```python
from build123d import *
from build123d.topology import SkipClean

# Parameters (mm, degrees)
SKETCH_1_R               = 5
SKETCH_1_R_2             = 3.5
EXTRUDE_1_DEPTH          = 2
EXTRUDE_2_DEPTH          = 2
CUT_EXTRUDE_1_DEPTH      = 61.539243471
CUT_EXTRUDE_1_DEPTH_BACK = 61.539243471
EXTRUDE_3_DEPTH          = 0.25
EXTRUDE_4_DEPTH          = 2
CUT_EXTRUDE_START        = 1
CUT_EXTRUDE_2_DEPTH      = 63.641007782
CUT_EXTRUDE_3_DEPTH      = 61.641007782
CUT_EXTRUDE_3_DEPTH_BACK = 61.641007782
SKETCH_8_R               = 0.706141664
EXTRUDE_5_DEPTH          = 4.5


with BuildPart() as part:
    # 草图1 → 凸台-拉伸1 (new, symmetric)
    with BuildSketch(Plane(origin=(0, 0, 0), x_dir=(1, 0, 0), z_dir=(0, 1, 0))):
        with Locations(Location((0, 0, 0), (0, 0, 270))):
            Circle(SKETCH_1_R)
        with Locations(Location((0, 0, 0), (0, 0, 270))):
            Circle(SKETCH_1_R_2, mode=Mode.SUBTRACT)
    extrude(amount=EXTRUDE_1_DEPTH, both=True)

    # 草图3 → 凸台-拉伸2 (add, symmetric)
    with BuildSketch(Plane(origin=(0, 0, 0), x_dir=(1, 0, 0), z_dir=(0, 1, 0))):
        with BuildLine():
            ThreePointArc((-4.530759254, -2.114762536), (-2.959942563, -6.862777701), (-2.534847218, -11.845789545))
            Line((-2.534847218, -11.845789545), (-3.308166283, -35.931035681))
            ThreePointArc((-3.308166283, -35.931035681), (-4.349252604, -47.119849682), (-6.737299363, -58.100316528))
            ThreePointArc((-6.737299363, -58.100316528), (0, -53), (6.737299363, -58.100316528))
            ThreePointArc((6.737299363, -58.100316528), (4.349252604, -47.119849682), (3.308166283, -35.931035681))
            Line((3.308166283, -35.931035681), (2.534847218, -11.845789545))
            ThreePointArc((2.534847218, -11.845789545), (2.959942563, -6.862777701), (4.530759254, -2.114762536))
            ThreePointArc((4.530759254, -2.114762536), (0, -5), (-4.530759254, -2.114762536))
        make_face()
        with BuildLine():
            Line((-7, -60), (7, -60))
            ThreePointArc((7, -60), (0, -53), (-7, -60))
        make_face()
    extrude(amount=EXTRUDE_2_DEPTH, both=True)

    # 草图4 → 切除-拉伸1 (cut, two sides: drawn at the far end of the back side and taken through both)
    with BuildSketch(Plane(origin=(0, 2, 0), x_dir=(1, 0, 0), z_dir=(0, 1, 0)).offset(-CUT_EXTRUDE_1_DEPTH_BACK)):
        with BuildLine():
            Line((-3, -60), (3, -60))
            ThreePointArc((3, -60), (0, -57), (-3, -60))
        make_face()
    extrude(amount=CUT_EXTRUDE_1_DEPTH + CUT_EXTRUDE_1_DEPTH_BACK, mode=Mode.SUBTRACT)

    # 草图5 → 凸台-拉伸3 (add, symmetric)
    with SkipClean():  # the faces are left unmerged after this step: merging them gives an invalid solid
        with BuildSketch(Plane(origin=(0, 2, 0), x_dir=(1, 0, 0), z_dir=(0, 1, 0))):
            with BuildLine():
                Line((-3, -60), (-7, -60))
                ThreePointArc((-7, -60), (0, -53), (7, -60))
                Line((7, -60), (3, -60))
                ThreePointArc((3, -60), (0, -57), (-3, -60))
            make_face()
        extrude_3 = extrude(amount=EXTRUDE_3_DEPTH, both=True)

    # 镜向1: 凸台-拉伸3 across plane
    with SkipClean():  # the faces are left unmerged after this step: merging them gives an invalid solid
        add(extrude_3.mirror(Plane.ZX))

    # 草图6 → 凸台-拉伸4 (add, symmetric)
    with BuildSketch(Plane(origin=(0, 0, 0), x_dir=(1, 0, 0), z_dir=(0, 1, 0))):
        with BuildLine():
            Line((-8.501136679, -55.801748406), (-8.501136679, -60))
            Line((-8.501136679, -60), (-7, -60))
            ThreePointArc((-7, -60), (-6.934013828, -59.041119283), (-6.737299363, -58.100316528))
            ThreePointArc((-6.737299363, -58.100316528), (-4.907121304, -50.347633667), (-3.749679969, -42.466391834))
            ThreePointArc((-3.749679969, -42.466391834), (-5.3686221, -49.403716977), (-8.501136679, -55.801748406))
        make_face()
        with BuildLine():
            Line((8.501136679, -60), (7, -60))
            ThreePointArc((7, -60), (6.934013828, -59.041119283), (6.737299363, -58.100316528))
            ThreePointArc((6.737299363, -58.100316528), (4.907121304, -50.347633667), (3.749679969, -42.466391834))
            ThreePointArc((3.749679969, -42.466391834), (5.3686221, -49.403716977), (8.501136679, -55.801748406))
            Line((8.501136679, -55.801748406), (8.501136679, -60))
        make_face()
    extrude(amount=EXTRUDE_4_DEPTH, both=True)

    # 草图7 → 切除-拉伸2 (cut)
    with BuildSketch(Plane(origin=(0, 0, 0), x_dir=(1, 0, 0), z_dir=(0, 1, 0)).offset(CUT_EXTRUDE_START)):
        with BuildLine():
            Line((-2.032181597, -10.971248009), (-2.792905901, -34.66422669))
            ThreePointArc((-2.792905901, -34.66422669), (0, -35.636501302), (2.792905901, -34.66422669))
            Line((2.792905901, -34.66422669), (2.032181597, -10.971248009))
            ThreePointArc((2.032181597, -10.971248009), (0, -9.921815328), (-2.032181597, -10.971248009))
        make_face()
    cut_extrude_2 = extrude(amount=CUT_EXTRUDE_2_DEPTH, mode=Mode.SUBTRACT)

    # 镜向2: 切除-拉伸2 across plane
    add(cut_extrude_2.mirror(Plane.ZX), mode=Mode.SUBTRACT)

    # 草图8 → 切除-拉伸3 (cut, two sides: drawn at the far end of the back side and taken through both)
    with BuildSketch(Plane.XY.offset(-CUT_EXTRUDE_3_DEPTH_BACK)):
        with Locations((-6.917679895, 0.156331749)):
            Circle(SKETCH_8_R)
        with Locations((6.917679895, 0.156331749)):
            Circle(SKETCH_8_R)
    extrude(amount=CUT_EXTRUDE_3_DEPTH + CUT_EXTRUDE_3_DEPTH_BACK, mode=Mode.SUBTRACT)

    # 草图11 → 凸台-拉伸5 (add)
    with BuildSketch(Plane(origin=(0, 2.25, 0), x_dir=(1, 0, 0), z_dir=(0, 1, 0))):
        with BuildLine():
            Line((8.501136679, -64.198251594), (8.501136679, -60))
            Line((8.501136679, -60), (3, -60))
            ThreePointArc((3, -60), (0, -63), (-3, -60))
            Line((-3, -60), (-8.501136679, -60))
            Line((-8.501136679, -60), (-8.501136679, -64.198251594))
            ThreePointArc((-8.501136679, -64.198251594), (-8.066557797, -64.898765683), (-7.650409709, -65.61038325))
            ThreePointArc((-7.650409709, -65.61038325), (0, -69.487105403), (7.650409709, -65.61038325))
            ThreePointArc((7.650409709, -65.61038325), (8.066557797, -64.898765683), (8.501136679, -64.198251594))
        make_face()
    extrude(amount=-EXTRUDE_5_DEPTH)


solid = part.part
```
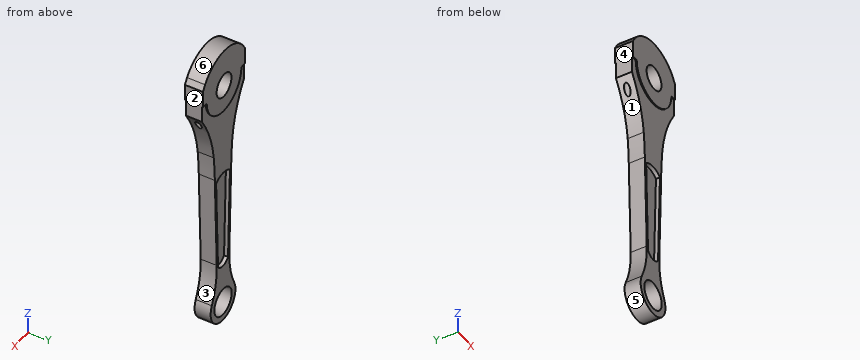
The model under review builds one solid part; all positions refer to its coordinate system, in mm. Face numbers are marked on the shaded views. A direction names the side the tool comes from. Give positions to 0.01 mm unless a question says otherwise; leave off trailing zeros. Write each loop counter-clockwise with the first axis right and the second up, starting at its lowest first coordinate (ties: lowest second). Pieces come first, ordered by that corner, then holes.
(1) To check wall thickness, follow L1, parallel to Z at x = 0.25, y = 1.35; L2, parallel to X at y = 1, z = 60; L3, parallel to X at y = -0.35, z = 0. State the ranges of each line that lie inside material, in increasing order.
(2) Tool access review of the marked faces 1, 2 and 3: name each direction out of +Z, -Z, +X, -X, +Y, -Y from which nothing blocks a thin tool from reaching the whole face with its end or side.
(3) Consider section D-D, the plane z = 41. Give the boundary of the cut face in (x, y), and give its area (3 significant figures).
(4) The part is to be moulded in two halves that separate along Z. For the marked faces 4, 5 and 6, say which applies: released by +Z, released by -Z, zero draft, split by the parting line, or undercut.
(5) Consider section B-B, the plane z = 0. Give the boundary of the cut face in (x, y), and give its area (3 significant figures).
(6) For P1, Ø3, axis at x = -0.5, z = 28.5, coming from the +Y side; P2, Ø1.3, axis at x = -6.92, y = 0.16, coming from the +Z side; P3, Ø1.6, axis at x = 7, y = 0, coming from the -Z side; P4, Ø5.5, axis at x = 0, z = 0, coming from the +Y side, all flat-tipped, find the tip position at first contact; note any pin that passes through.
(7) Consider section A-A, the plane x = 0. Give the boundary of the cut face in (y, z).
(8) Consider section C-C, the plane z = 13.5. Give the boundary of the cut face in (x, y).
Returned:
1. L1: z = -4.99 to -3.49, 3.49 to 9.93, 35.63 to 57.01, 62.99 to 69.48
1. L2: x = -8.5 to -3, 3 to 8.5
1. L3: x = -5 to -3.5, 3.5 to 5
2. face 1: -X, +Y, -Y
2. face 2: +Z, -Z, +X, +Y, -Y
2. face 3: +X, +Y, -Y
3. outline: (-3.61, -2) - (3.61, -2) - (3.61, 2) - (-3.61, 2) - close
3. area: 28.9 mm2
4. face 4: zero draft
4. face 5: undercut
4. face 6: released by +Z
5. outline: (-5, -2) - (-3.5, -2) - (-3.5, 2) - (-5, 2) - close; (3.5, -2) - (5, -2) - (5, 2) - (3.5, 2) - close
5. area: 12.0 mm2
6. P1: stops at y = 1
6. P2: stops at z = 67.12
6. P3: stops at z = 51.5
6. P4: passes through
7. outline: (-2.25, 53) - (-2, 53) - (-2, 35.64) - (-1, 35.64) - (-1, 9.92) - (-2, 9.92) - (-2, 3.5) - (2, 3.5) - (2, 9.92) - (1, 9.92) - (1, 35.64) - (2, 35.64) - (2, 53) - (2.25, 53) - (2.25, 57) - (-2.25, 57) - close; (-2.25, 63) - (2.25, 63) - (2.25, 69.49) - (-2.25, 69.49) - close; (-2, -5) - (2, -5) - (2, -3.5) - (-2, -3.5) - close
8. outline: (-2.59, -2) - (-2.11, -2) - (-2.11, -1) - (2.11, -1) - (2.11, -2) - (2.59, -2) - (2.59, 2) - (2.11, 2) - (2.11, 1) - (-2.11, 1) - (-2.11, 2) - (-2.59, 2) - close
